Geometry: see drawing. Coordinates: mm, zero at the bounding-box minimum. A direction names the side the tool comes from. Round coordinates to 2 decimals unless told otherwise and drop trailing zeros. Order: outer loops, then holes, each group sorted by start corner. A loop starts at its lowest first (then second) coordinate and runs counter-clockwise, first axis right, second up. Notation, with made-up numbers: (-13, 39.25) -> (21, 39.25) arc R28 ccw to (21, 57.25) -> close; hole circle Ø10 at (43, -40). An arc over 180 degrees is marked (long way). Use a Markdown table: item, result.
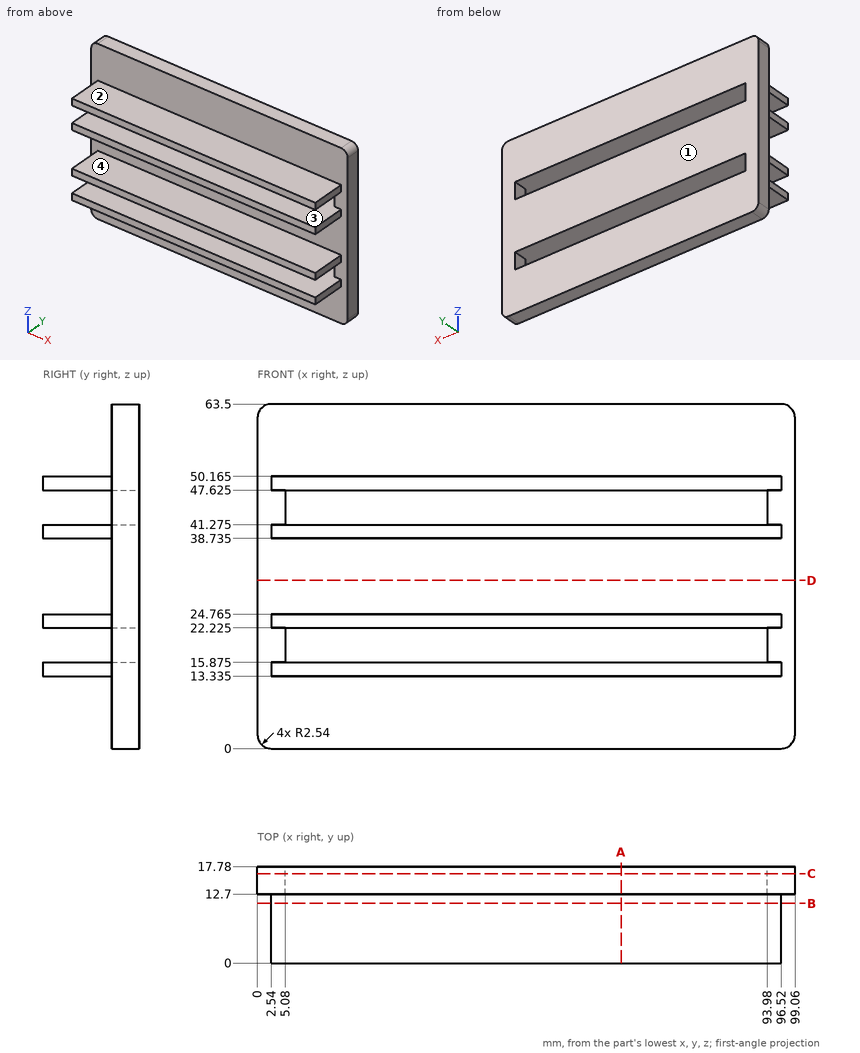
1) Draft query along X for the marked faces 3 and 4. Return one class per face: released by +X, released by -X, zero draft, split by the parting line, or undercut.
Answer key:
| item | result |
|---|---|
| face 3 | undercut |
| face 4 | zero draft |
2) Cut plane D-D on z = 31. Return loops of the section in (x, y), and give its area (3 significant figures).
Answer key:
| item | result |
|---|---|
| outline | (0, 12.7) -> (99.06, 12.7) -> (99.06, 17.78) -> (0, 17.78) -> close |
| area | 503 mm^2 |
3) Contact query for flat-ended pins moving along their axis: P1, Ø5, axis at x = 80.5, z = 54.5, coming from the -Y side; P2, Ø4, axis at x = 69.5, y = 6.5, coming from the -Z side (3 decimals); P3, Ø3, axis at y = 9, z = 14, coming from the +X side. Output: stop coordinate, or through.
Answer key:
| item | result |
|---|---|
| P1 | stops at y = 12.7 |
| P2 | stops at z = 13.335 |
| P3 | stops at x = 96.52 |
4) Cut plane B-B on y = 11. Return loops of the section in (x, z) (3 decimals), and give its area (3 significant figures).
Answer key:
| item | result |
|---|---|
| outline | (2.54, 13.335) -> (96.52, 13.335) -> (96.52, 15.875) -> (2.54, 15.875) -> close; (2.54, 22.225) -> (96.52, 22.225) -> (96.52, 24.765) -> (2.54, 24.765) -> close; (2.54, 38.735) -> (96.52, 38.735) -> (96.52, 41.275) -> (2.54, 41.275) -> close; (2.54, 47.625) -> (96.52, 47.625) -> (96.52, 50.165) -> (2.54, 50.165) -> close |
| area | 955 mm^2 |
5) Set-up query: the marked faces 1 and 2. Return all of +Z, -Z, +X, -X, +Y, -Y with unobstructed straight access to the full face (end or side cutting, diameter ignored); none if empty.
Answer key:
| item | result |
|---|---|
| face 1 | +Z, -Z, +X, -X, +Y |
| face 2 | +Z, +X, -X, -Y |
6) Ray query, probe 1 along Z at (x, y) = (15.5, 5.25) (3 decimals); probe 2 along Z at (x, y) = (91.5, 16.5) (3 decimals); probe 3 along X at (y, z) = (13.5, 21.5). Return the intervals inside material, ascending.
Answer key:
| item | result |
|---|---|
| probe 1 | z = 13.335 to 15.875, 22.225 to 24.765, 38.735 to 41.275, 47.625 to 50.165 |
| probe 2 | z = 0 to 15.875, 22.225 to 41.275, 47.625 to 63.5 |
| probe 3 | x = 0 to 5.08, 93.98 to 99.06 |
7) Cut plane C-C on y = 16.5. Return loops of the section in (x, z) (3 decimals).
Answer key:
| item | result |
|---|---|
| outline | (0, 2.54) arc R2.54 ccw to (2.54, 0) -> (96.52, 0) arc R2.54 ccw to (99.06, 2.54) -> (99.06, 60.96) arc R2.54 ccw to (96.52, 63.5) -> (2.54, 63.5) arc R2.54 ccw to (0, 60.96) -> close; hole (5.08, 15.875) -> (93.98, 15.875) -> (93.98, 22.225) -> (5.08, 22.225) -> close; hole (5.08, 41.275) -> (93.98, 41.275) -> (93.98, 47.625) -> (5.08, 47.625) -> close |
8) Cut plane A-A on x = 67. Return loops of the section in (y, z) (3 decimals), and give its area (3 significant figures).
Answer key:
| item | result |
|---|---|
| outline | (0, 13.335) -> (12.7, 13.335) -> (12.7, 0) -> (17.78, 0) -> (17.78, 15.875) -> (0, 15.875) -> close; (0, 22.225) -> (17.78, 22.225) -> (17.78, 41.275) -> (0, 41.275) -> (0, 38.735) -> (12.7, 38.735) -> (12.7, 24.765) -> (0, 24.765) -> close; (0, 47.625) -> (17.78, 47.625) -> (17.78, 63.5) -> (12.7, 63.5) -> (12.7, 50.165) -> (0, 50.165) -> close |
| area | 387 mm^2 |
